Design review of the part built by this model. Coordinates are the model's own, in mm. A direction names the side the tool comes from. Round coordinates to 2 decimals unless told otherwise and drop trailing zeros. Order: outer loops, then holes, each group sorted by start corner. A loop starts at its lowest first (then second) coordinate and runs counter-clockwise, first axis right, second up. Notation, with made-up numbers: (40.5, 36) - (84.5, 36) arc R26 cw to (84.5, 66) - close; hole circle Ø4 at (34, 12). An arc over 180 degrees is marked (long way). Write item = value, one per line.
from build123d import *

# Parameters (mm, degrees)
FILLET1_R          = 2
SKETCH2_R          = 24
CUT_EXTRUDE1_DEPTH = 70.225501822


with BuildPart() as part:
    # Sketch1 → Revolve1 (revolve)
    with BuildSketch(Plane.XY, mode=Mode.PRIVATE) as revolve1_sk:
        Polygon((-11.65, -39.8), (11.65, -39.8), (13.5, -29.6), (15.75, -29.6), (15.75, -23.6), (4.25, -20.75), (4.25, -17), (20.15, -15.75), (20.15, -10.05), (-20.15, -10.05), (-20.15, -15.75), (-4.25, -17), (-4.25, -20.75), (-15.75, -23.6), (-15.75, -29.6), (-13.5, -29.6), align=None)
    revolve(revolve1_sk.sketch.rotate(Axis((0, 0, 0), (1, 0, 0)), 270), axis=Axis((0, 0, 0), (1, 0, 0)))

    # Fillet1
    fillet1_edges = [part.edges().sort_by_distance(p)[0] for p in [
        (11.65, 0, -39.8),
        (-11.65, 0, -39.8),
        (-4.25, 0, -20.75),
        (-4.25, 0, -17),
        (-20.15, 0, -15.75),
        (20.15, 0, -15.75),
        (4.25, 0, -17),
        (4.25, 0, -20.75),
    ]]
    fillet(fillet1_edges, radius=FILLET1_R)

    # Sketch2 → Cut-Extrude1 (cut, through all)
    with BuildSketch(Plane(origin=(20.15, 0, 0), x_dir=(0, 0, -1), z_dir=(1, 0, 0))):
        Circle(SKETCH2_R)
    extrude(amount=-CUT_EXTRUDE1_DEPTH, mode=Mode.SUBTRACT)


solid = part.part
1) We need section A-A on x = -4. Write out the cut boundary in (y, z), and give its area (3 significant figures).
Findings:
outline = circle Ø79.6 at (0, 0); hole circle Ø48 at (0, 0)
area = 3,170 mm^2
2) For faces 1 (the cylindrical face through (-14.6, 28.9, -6.4)), 2 (the cylindrical face through (0.221, 1.055, 23.977)), 3 (the cylindrical face through (14.6, 28.9, -6.4)), list the 3-axis set-ups (+Z, -Z, +X, -X, +Y, -Y) from which the entire face can be reached by the end or side of a thin tool; tool diameter is ignored.
Findings:
face_1 = -X
face_2 = +X, -X
face_3 = +X
3) To check wall thickness, follow L1, parallel to Y at x = 8, z = 0; L2, parallel to Z at x = -8, y = -5; L3, parallel to Z at x = 10.5, y = 26.5. State the ranges of each line that lie inside material, in increasing order. Write a range as from..to.
Findings:
L1 = -39.8..-24, 24..39.8
L2 = -39.48..-23.47, 23.47..39.48
L3 = -29.6..29.6
4) Clearance check with flat-ended pins moving along their axes: pin 1 Ø5 at (y, z) = (-14, -27) entering from +X; pin 2 Ø5 at (x, z) = (7, 2) entering from +Y; pin 3 Ø5 at (y, z) = (17.5, -31) entering from +X; pin 4 Ø5 at (x, y) = (10, 30.5) entering from -Z. State where each tip first meets the part, or that it passes through.
Findings:
pin_1 = 15.75
pin_2 = 39.8
pin_3 = 12.87
pin_4 = -28.28
